Could you check a few things on this drawing? It's one solid part, dimensions in mm from its lowest x, y, z. A direction names the side the tool comes from. Give positions to 0.01 mm unless a question says otherwise; leave off trailing zeros. Order: outer loops, then holes, each group sorted by start corner. A loop starts at its lowest first (then second) coordinate and runs counter-clockwise, first axis right, second up. Notation, with made-up numbers: (77, 54) -> (97, 54) arc R22 cw to (97, 89) -> close; hole circle Ø5 at (-25.75, -18). An arc over 180 degrees is marked (long way). Answer as a JSON object with one key per item and string values.
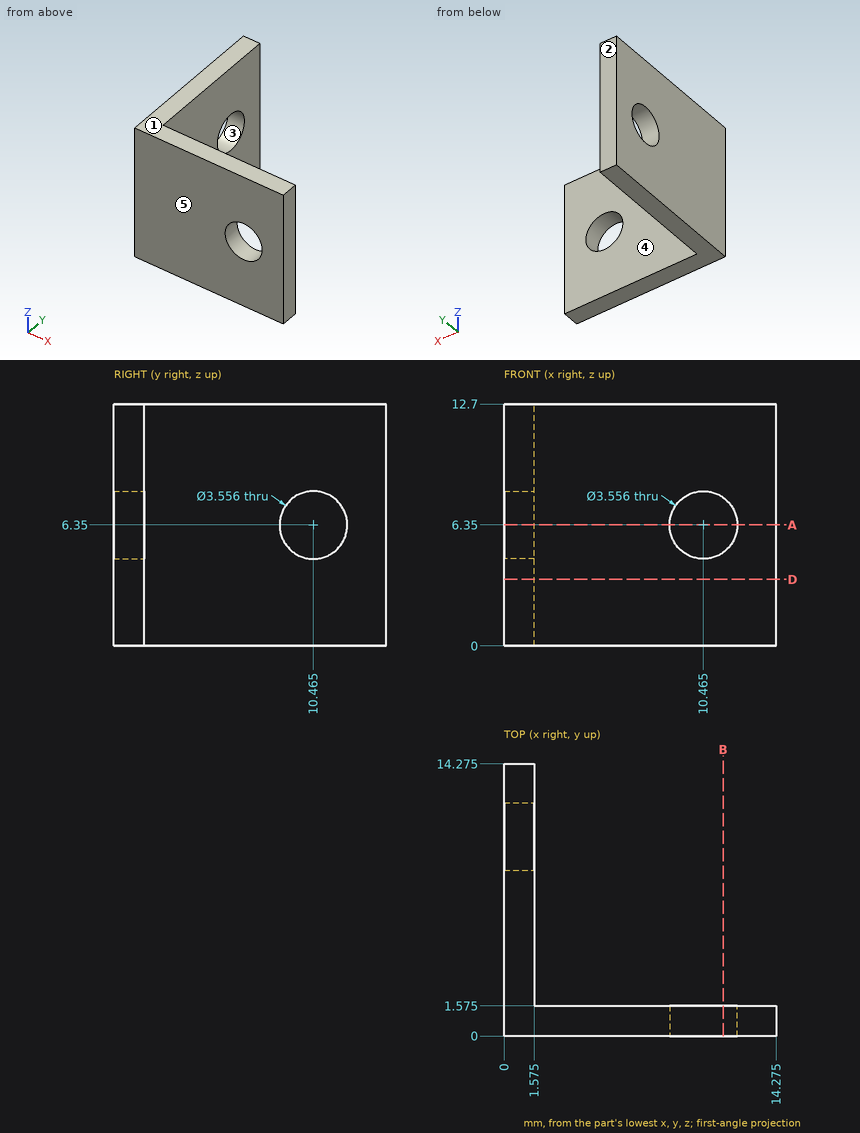
1. If we mould it in two halves opening along Z, with no side actions, what happens to the marked faces 1, 2 and 3? For each: +Z half, -Z half, draft (parallel to the pull), parting line (faces both ways), or undercut.
Worked answers:
{"face 1": "+Z half", "face 2": "draft", "face 3": "undercut"}
2. Please list where these lines run through material, in increasing order: L1, parallel to X at y = 7, z = 3 (1 decimal); L2, parallel to Y at x = 0.6, z = 6.35 (1 decimal).
Worked answers:
{"L1": "0 to 1.6", "L2": "0 to 8.7, 12.2 to 14.3"}
3. If we section it at D-D on z = 3.5: Please give me the cut outline in (x, y) (1 decimal), then the cut area to 3 significant figures.
Worked answers:
{"outline": "(0, 0) -> (14.3, 0) -> (14.3, 1.6) -> (1.6, 1.6) -> (1.6, 14.3) -> (0, 14.3) -> close", "area": "42.5 mm²"}
4. If we section it at B-B on x = 11.5: Please give me the cut outline in (y, z) (1 decimal).
Worked answers:
{"outline": "(0, 0) -> (1.6, 0) -> (1.6, 4.9) -> (0, 4.9) -> close; (0, 7.8) -> (1.6, 7.8) -> (1.6, 12.7) -> (0, 12.7) -> close"}
5. If we section it at A-A on z = 6.35: Please give me the cut outline in (x, y) (1 decimal), then the cut area to 3 significant figures.
Worked answers:
{"outline": "(0, 0) -> (8.7, 0) -> (8.7, 1.6) -> (1.6, 1.6) -> (1.6, 8.7) -> (0, 8.7) -> close; (0, 12.2) -> (1.6, 12.2) -> (1.6, 14.3) -> (0, 14.3) -> close; (12.2, 0) -> (14.3, 0) -> (14.3, 1.6) -> (12.2, 1.6) -> close", "area": "31.3 mm²"}
6. For the marked faces 4 and 5, which set-ups out of +Z, -Z, +X, -X, +Y, -Y let a thin tool reach every point of the face, with its end or its side?
Worked answers:
{"face 4": "+Z, -Z, +X, +Y", "face 5": "+Z, -Z, +X, -X, -Y"}
7. Will this pin go through, and if not, where does the flat tip stop? pin 1 Ø6 at (y, z) = (8.5, 10) entering from +X (3 decimals).
Worked answers:
{"pin 1": "x = 1.575"}
